Build history of the part. All positions in model axes, mm. A direction names the side the tool comes from. Round coordinates to 2 decimals unless told otherwise and drop trailing zeros. Write each loop counter-clockwise with the first axis right and the second up, starting at its lowest first coordinate (ties: lowest second). Pieces come first, ordered by that corner, then holes. Notation, with made-up numbers: (24.5, 38.5) -> (34.5, 38.5) arc R11 cw to (34.5, 45.5) -> close; hole circle Ø3 at (19, 65.25). An arc over 180 degrees is marked (long way). Return JSON: item names as keys, results as strings.
from build123d import *

# Parameters (mm, degrees)
F0_W     = 107.320446521
F0_H     = 112.5355064869
F1_DEPTH = 25.4
F2_R     = 10
F2_W     = 44.1350700906
F2_H     = 10
F3_DEPTH = 107.321446621
F4_R     = 10
F5_DEPTH = 25.4010001


with BuildPart() as f1:
    # F0 (on Top) → F1 (new body)
    with BuildSketch(Plane.XY):
        with Locations((-0.9606685489, -0.4117153585)):
            Rectangle(F0_W, F0_H)
        with BuildLine():
            Line((-13.9983193949, -30.3296931088), (-36.7798954248, -29.5062605292))
            add(Edge.make_bspline(
                [(-36.7798954248, -29.5062605292), (-37.0737623342, -22.3038153757), (-37.7074826154, -6.7718333039), (-11.6101098174, 5.4940779058), (11.5229911211, 16.1858602813), (8.1523007319, 29.4068529306), (6.5874438733, 35.5447530746)],
                knots=[0, 0, 0, 0, 0.2420361752, 0.5219479572, 0.7780623755, 1, 1, 1, 1], degree=3))
            Line((6.5874438733, 35.5447530746), (24.1539627314, 39.6619029343))
            add(Edge.make_bspline(
                [(-13.9983193949, -30.3296931088), (-12.7174517336, -25.9697019043), (-10.0863175924, -17.0134903766), (5.2905439896, -15.0083142094), (21.4625052751, -3.7589083207), (31.1936947319, 13.367953183), (26.6480589275, 30.3462585247), (24.1539627314, 39.6619029343)],
                knots=[0, 0, 0, 0, 0.1678735533, 0.3448426804, 0.5534704946, 0.7549985109, 1, 1, 1, 1], degree=3))
        make_face(mode=Mode.SUBTRACT)
    extrude(amount=F1_DEPTH)

    # F2 (on face) → F3 (cut, through all)
    with BuildSketch(Plane.YZ.offset(52.6995547116)):
        with Locations((-32.3753028454, 12.2389346361)):
            Circle(F2_R)
        with Locations((35.833440075, 14.731259873)):
            Rectangle(F2_W, F2_H)
    extrude(amount=-F3_DEPTH, mode=Mode.SUBTRACT)

    # F4 (on face) → F5 (cut, through all)
    with BuildSketch(Plane.XY.offset(25.4)):
        with Locations((-5.7272729464, 24.6272739023)):
            Circle(F4_R)
    extrude(amount=-F5_DEPTH, mode=Mode.SUBTRACT)


solid = f1.part
Q1. 3-axis set-ups, long thin cutter, end or side, ignore diameter. For faces 4 (the flat face through (0, 35, 9.731)), 5 (the flat face through (15.248, 37.575, 22.526)), 6 (the flat face through (-2, 13, 25.4)): which of +Z, -Z, +X, -X, +Y, -Y reach the whole face in a straight line?
Verdict:
{"face 4": "+X, -X, +Y", "face 5": "+Z, -Z", "face 6": "+Z, +X, -X, +Y, -Y"}
Q2. Wall check: L1, parallel to Z at x = 48, y = 38.5; L2, parallel to Y at x = -9, z = 12; L3, parallel to Y at x = -25, z = 4.5. Give the ranges that are in metal, low to high.
Verdict:
{"L1": "z = 0 to 9.73, 19.73 to 25.4", "L2": "y = -56.68 to -42.37, -22.38 to -19.53, 6.68 to 13.77", "L3": "y = -56.68 to -38.71, -1.48 to 55.86"}
Q3. Saw through at C-C on x = 20.5. Count the separate pieces of the cut face and the enclosed holes in it, then the cut area to 3 significant figures.
Verdict:
{"separate pieces": "3", "enclosed holes": "1", "area": "1,320 mm²"}
Q4. Saw through at A-A on y = 44. List the corners of the cut face in (x, z).
Verdict:
{"outline": "(-54.62, 0) -> (52.7, 0) -> (52.7, 9.73) -> (-54.62, 9.73) -> close; (-54.62, 19.73) -> (52.7, 19.73) -> (52.7, 25.4) -> (-54.62, 25.4) -> close"}
Q5. Two-plate mould, pull along X, no slides. Class faces 1 (the flat face through (-25.23, -29.924, 1.311)), 2 (the cylindrical face through (-0.209, -42.366, 12.679)), 3 (the flat face through (52.7, -1, 13)): +X half, -X half, draft (parallel to the pull), parting line (faces both ways), or undercut.
Verdict:
{"face 1": "undercut", "face 2": "draft", "face 3": "+X half"}
Q6. Saw through at B-B on x = 38. List the corners of the cut face in (y, z), then the cut area to 3 significant figures.
Verdict:
{"outline": "(-56.68, 0) -> (55.86, 0) -> (55.86, 9.73) -> (13.77, 9.73) -> (13.77, 19.73) -> (55.86, 19.73) -> (55.86, 25.4) -> (-56.68, 25.4) -> close; hole circle Ø20 at (-32.38, 12.24)", "area": "2,120 mm²"}
Q7. Pin check, flat tip, straight feed: pin 1 Ø5 at (x, z) = (-27.5, 17) entering from +Y. Stop position of the tip, or through.
Verdict:
{"pin 1": "stops at y = 13.77"}
